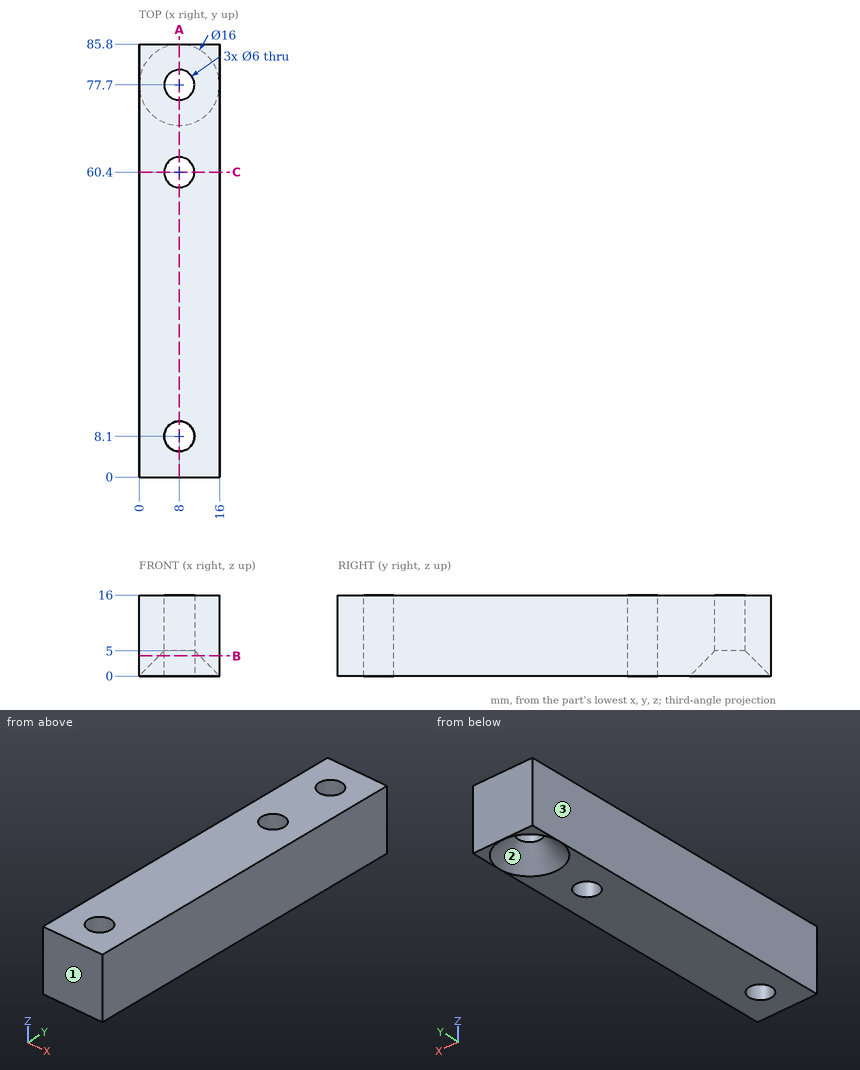
Could you check a few things on this drawing? It's one solid part, dimensions in mm from its lowest x, y, z. Round coordinates to 2 decimals unless told otherwise and drop trailing zeros. Order: outer loops, then holes, each group sorted by start corner. A loop starts at its lowest first (then second) coordinate and runs counter-clockwise, first axis right, second up.
Q1. Imagine slicing it at C-C, the plane y = 60.4. List the corners of the cut face in (x, z) for me.
Geometry says:
outline: (0, 0) - (5, 0) - (5, 16) - (0, 16) - close; (11, 0) - (16, 0) - (16, 16) - (11, 16) - close
Q2. Imagine slicing it at A-A, the plane x = 8. List the corners of the cut face in (y, z) for me.
Geometry says:
outline: (0, 0) - (5.1, 0) - (5.1, 16) - (0, 16) - close; (11.1, 0) - (57.4, 0) - (57.4, 16) - (11.1, 16) - close; (63.4, 0) - (69.7, 0) - (74.7, 5) - (74.7, 16) - (63.4, 16) - close; (80.7, 5) - (85.7, 0) - (85.8, 0) - (85.8, 16) - (80.7, 16) - close
Q3. Imagine slicing it at B-B, the plane z = 4. List the corners of the cut face in (x, y) for me.
Geometry says:
outline: (0, 0) - (16, 0) - (16, 85.8) - (0, 85.8) - close; hole circle Ø8 at (8, 77.7); hole circle Ø6 at (8, 8.1); hole circle Ø6 at (8, 60.4)
Q4. Please list where these lines run through material, in increasing order: probe 1 along Y at (x, z) = (8, 8.25); probe 2 along X at (y, z) = (77.7, 8); probe 3 along Y at (x, z) = (10.5, 10.75).
Geometry says:
probe 1: y = 0 to 5.1, 11.1 to 57.4, 63.4 to 74.7, 80.7 to 85.8
probe 2: x = 0 to 5, 11 to 16
probe 3: y = 0 to 6.44, 9.76 to 58.74, 62.06 to 76.04, 79.36 to 85.8
Q5. I'm going to push flat-ended pins straight in: P1, Ø3, axis at y = 56.5, z = 2, coming from the -X side; P2, Ø9.5, axis at x = 8, y = 77.7, coming from the -Z side. Where does each tip first touch, or does it pass through?
Geometry says:
P1: stops at x = 0
P2: stops at z = 3.25
Q6. Thinking about a two-plate mould opening in X: for the marked faces 1, 2 and 3, which applies, released by +X, released by -X, zero draft, split by the parting line, or undercut?
Geometry says:
face 1: zero draft
face 2: undercut
face 3: released by -X
